```python
from build123d import *

# Parameters (mm, degrees)
BOSS_EXTRUDE1_DEPTH = 4


with BuildPart() as part:
    # Sketch1 → Boss-Extrude1 (new body)
    with BuildSketch(Plane.XY):
        with BuildLine():
            Line((0, 13), (4.5, 13))
            Line((4.5, 13), (4.5, 17))
            Line((4.5, 17), (8.5, 17))
            Line((8.5, 17), (8.5, 13))
            Line((8.5, 13), (13, 13))
            Line((13, 13), (13, 11.5))
            add(Edge.make_bspline(
                [(1.5, 0), (2.52035849, 4.950366231), (6.473986228, 10.017019138), (13, 11.5)],
                knots=[0, 0, 0, 0, 1, 1, 1, 1], degree=3))
            Line((1.5, 0), (0, 0))
            Line((0, 0), (0, 4.987852908))
            Line((0, 4.987852908), (-4, 4.987852908))
            Line((-4, 4.987852908), (-4, 8.987852908))
            Line((-4, 8.987852908), (0, 8.987852908))
            Line((0, 8.987852908), (0, 13))
        make_face()
    extrude(amount=BOSS_EXTRUDE1_DEPTH)


solid = part.part
```
Input: part model. Units: mm. Frame: model coordinates. A direction names the side the tool comes from. Give positions to 0.01 mm unless a question says otherwise; leave off trailing zeros. Loops run counter-clockwise (first coordinate to the right, second up) from the corner with the lowest first, then second, coordinate; pieces in that order, holes last. Notation, with made-up numbers: M -1,-1 L 32,-1 A23 cw 32,33 Z; hole C 66,-17.75 d4. An arc over 180 degrees is marked long. Answer as CSV lines item,"result". Start each with the question number.
1. Section A-A on y = 12.25. Return loops of the section in (x, z).
2. Pin query (flat end, axial travel): P1, Ø1.2, axis at x = -3, z = 3, coming from the -Y side; P2, Ø2, axis at y = 3, z = 3.5, coming from the -X side; P3, Ø1.2, axis at x = 2, z = 2, coming from the +Y side. Return the tip coordinate at first contact, or that it passes through.
3. Section B-B on x = -0.75. Return loops of the section in (y, z), plus the area to 3 significant figures.
4. Reachability of faces 1 (the face through (8.5, 15, 2)), 2 (the face through (-4, 7, 2)), 3 (the face through (6, 17, 2)), 4 (the face through (2, 13, 2)), 5 (the face through (0, 2, 2)) from +Z, -Z, +X, -X, +Y, -Y: full face, straight path, thin tool, end or side. Return the list, or none.
5. Line query: L1, parallel to X at y = 16, z = 2.1; L2, parallel to Y at x = -0.25, z = 1.55; L3, parallel to Y at x = 1, z = 0.95. Output: solid intervals per line, ascending.
Computed values:
1,outline,"M 0,0 L 13,0 L 13,4 L 0,4 Z"
2,P1,"stops at y = 4.99"
2,P2,"stops at x = 0"
2,P3,"stops at y = 13"
3,outline,"M 4.99,0 L 8.99,0 L 8.99,4 L 4.99,4 Z"
3,area,"16.0 mm²"
4,face 1,"+Z, -Z, +X, +Y"
4,face 2,"+Z, -Z, -X, +Y, -Y"
4,face 3,"+Z, -Z, +X, -X, +Y"
4,face 4,"+Z, -Z, -X, +Y"
4,face 5,"+Z, -Z, -X, -Y"
5,L1,"x = 4.5 to 8.5"
5,L2,"y = 4.99 to 8.99"
5,L3,"y = 0 to 13"
